Verification items for the finished model (mm, model axes). Round coordinates to 2 decimals unless told otherwise and drop trailing zeros. Order: outer loops, then holes, each group sorted by start corner. A loop starts at its lowest first (then second) coordinate and runs counter-clockwise, first axis right, second up. Notation, with made-up numbers: M 58.25,47 L 86.25,47 A16 ccw 86.25,78 Z; hole C 15,42 d6. An arc over 180 degrees is marked long. Use one line per item in the form item = value. Start each with the question number.
Item 1: Cross-section at D-D on x = -25. Enter the section's corners in (y, z), then the cut area to 3 significant figures.
Item 2: Cross-section at A-A on x = 33. Enter the section's corners in (y, z).
Item 3: Release check for a two-part mould opening along Z. For faces 1 (the flat face through (-55, -2, -1)), 2 (the flat face through (-3, -2, -40)), 3 (the cylindrical face through (48.24, -2.465, 17.483)) record: +Z half, -Z half, draft (parallel to the pull), parting line (faces both ways), or undercut.
Item 4: Cross-section at B-B on x = 17.5. Enter the section's corners in (y, z), then the cut area to 3 significant figures.
Item 5: Cross-section at C-C on y = -2.8. Count the separate pieces of the cut face and the enclosed holes in it, then the cut area to 3 significant figures.
Item 6: Thickness scan on probe 1 along Z at (x, y) = (-25, -4); probe 2 along Z at (x, y) = (17.5, -2.1); probe 3 along Z at (x, y) = (-26, -1.1). Record the ranges inside material, lowest first. Write a range as [from, to].
from build123d import *

# Parameters (mm, degrees)
F0_W     = 110
F0_H     = 80
F0_R     = 2
F0_R_2   = 4.5
F0_R_3   = 3
F1_DEPTH = 5
F2_SIZE  = 4.5
F3_SIZE  = 4.5


with BuildPart() as f1:
    # F0 (on Front) → F1 (new body)
    with BuildSketch(Plane.XZ):
        Rectangle(F0_W, F0_H)
        with Locations((-25, -18.5)):
            Circle(F0_R, mode=Mode.SUBTRACT)
        with Locations((17.5, -15.5)):
            Circle(F0_R, mode=Mode.SUBTRACT)
        with Locations((48.5, -15.5)):
            Circle(F0_R, mode=Mode.SUBTRACT)
        with Locations((-25, 0)):
            Circle(F0_R_2, mode=Mode.SUBTRACT)
        with Locations((-25, 18.5)):
            Circle(F0_R, mode=Mode.SUBTRACT)
        with Locations((17.5, 15.5)):
            Circle(F0_R, mode=Mode.SUBTRACT)
        with Locations((33, 0)):
            Circle(F0_R_3, mode=Mode.SUBTRACT)
        with Locations((48.5, 15.5)):
            Circle(F0_R, mode=Mode.SUBTRACT)
    extrude(amount=F1_DEPTH)

    # F2
    f2_edges = [f1.edges().sort_by_distance(p)[0] for p in [
        (55, -2.5, 40),
    ]]
    chamfer(f2_edges, length=F2_SIZE)

    # F3
    f3_edges = [f1.edges().sort_by_distance(p)[0] for p in [
        (55, -2.5, -40),
    ]]
    chamfer(f3_edges, length=F3_SIZE)


solid = f1.part
Output values:
q1.outline = M -5,-40 L 0,-40 L 0,-20.5 L -5,-20.5 Z; M -5,-16.5 L 0,-16.5 L 0,-4.5 L -5,-4.5 Z; M -5,4.5 L 0,4.5 L 0,16.5 L -5,16.5 Z; M -5,20.5 L 0,20.5 L 0,40 L -5,40 Z
q1.area = 315 mm2
q2.outline = M -5,-40 L 0,-40 L 0,-3 L -5,-3 Z; M -5,3 L 0,3 L 0,40 L -5,40 Z
q3.face_1 = draft
q3.face_2 = -Z half
q3.face_3 = undercut
q4.outline = M -5,-40 L 0,-40 L 0,-17.5 L -5,-17.5 Z; M -5,-13.5 L 0,-13.5 L 0,13.5 L -5,13.5 Z; M -5,17.5 L 0,17.5 L 0,40 L -5,40 Z
q4.area = 360 mm2
q5.separate_pieces = 1
q5.enclosed_holes = 8
q5.area = 8,610 mm2
q6.probe_1 = [-40, -20.5], [-16.5, -4.5], [4.5, 16.5], [20.5, 40]
q6.probe_2 = [-40, -17.5], [-13.5, 13.5], [17.5, 40]
q6.probe_3 = [-40, -20.23], [-16.77, -4.39], [4.39, 16.77], [20.23, 40]
